from build123d import *
from build123d import SkipClean  # not in build123d's __all__

# Parameters (mm, degrees)
F1_DEPTH      = 2
F0_W          = 5.54
F0_H          = 25
F0_W_2        = 1.9
F0_W_3        = 2.5
F0_H_2        = 2.5
F2_DEPTH      = 5
F3_DEPTH      = 5
F4_DEPTH      = 7
F5_SIZE       = 7
F8_DEPTH      = 2
F9_SIZE       = 1.5
F10_SIZE      = 1.5
F11_SIZE      = 1.5
F12_R         = 8
F13_R         = 2
F14_T4_DEPTH  = 20.4300979278
F14_T10_DEPTH = 20.4300979278


# Not quite as in the source:
# - a fillet or chamfer that OpenCascade refuses, or shapes differently, is made with other operations: its cross-section is extruded or revolved along the edge and cut away or added
# - ends of sketch curves that miss each other by under 0.0002 mm in the source are joined
# - a feature names something its author has since deleted; it is built from what else it names


with BuildPart() as f1:
    # F0 (on Front) → F1 (new body)
    with BuildSketch(Plane.XZ):
        with BuildLine():
            Line((-25, 38.2831491688), (-4.67, 38.2831491688))
            Line((-4.67, 38.2831491688), (-4.67, 63.2831491688))
            Line((-4.67, 63.2831491688), (-12.45, 63.2831491688))
            Line((-12.45, 63.2831491688), (-12.45, 58.8677023414))
            ThreePointArc((-12.45, 58.8677023414), (-7.0483053281, 56.3311217715), (-4.85, 50.7831491688))
            ThreePointArc((-4.85, 50.7831491688), (-18.4979726027, 44.8814544969), (-13.45, 58.8677023414))
            Line((-13.45, 58.8677023414), (-13.45, 63.2831491688))
            Line((-13.45, 63.2831491688), (-25, 63.2831491688))
            Line((-25, 63.2831491688), (-25, 38.2831491688))
        make_face()
    extrude(amount=F1_DEPTH)



with BuildPart() as f1b:
    # F0 (on Front) → F1, piece 2 (new body)
    with BuildSketch(Plane.XZ):
        with BuildLine():
            Line((4.67, 38.2831491688), (25, 38.2831491688))
            Line((25, 38.2831491688), (25, 63.2831491688))
            Line((25, 63.2831491688), (13.45, 63.2831491688))
            Line((13.45, 63.2831491688), (13.45, 58.8677023414))
            ThreePointArc((13.45, 58.8677023414), (18.8516946719, 56.3311217715), (21.05, 50.7831491688))
            ThreePointArc((21.05, 50.7831491688), (7.4020273973, 44.8814544969), (12.45, 58.8677023414))
            Line((12.45, 58.8677023414), (12.45, 63.2831491688))
            Line((12.45, 63.2831491688), (4.67, 63.2831491688))
            Line((4.67, 63.2831491688), (4.67, 38.2831491688))
        make_face()
    extrude(amount=F1_DEPTH)


with BuildPart() as f1c:
    # F0 (on Front) → F1, piece 3 (new body)
    with BuildSketch(Plane.XZ):
        with Locations((0, 50.7831491688)):
            Rectangle(F0_W, F0_H)
        Polygon((2.77, -9.5068508312), (2.77, 38.2831491688), (-2.77, 38.2831491688), (-2.77, -9.5068508312), (-1.5, -9.5068508312), (-1.5, -0.9968508312), (1.5, -0.9968508312), (1.5, -9.5068508312), align=None)
    extrude(amount=F1_DEPTH)


with BuildPart() as f1_1:
    add(f1.part, clean=False)

    add(f1b.part)  # F2 merges F1b

    add(f1c.part)  # F2 merges F1c
    # F0 (on Front) → F2 (join)
    with BuildSketch(Plane.XZ):
        Polygon((-2.77, -9.5068508312), (-2.77, 38.2831491688), (-4.67, 38.2831491688), (-4.67, 0), (-4.67, -7.0068508312), (-4.67, -9.5068508312), align=None)
        Polygon((4.67, -7.0068508312), (4.67, 38.2831491688), (2.77, 38.2831491688), (2.77, -9.5068508312), (4.67, -9.5068508312), align=None)
        with Locations((3.72, 50.7831491688)):
            Rectangle(F0_W_2, F0_H)
        with Locations((-3.72, 50.7831491688)):
            Rectangle(F0_W_2, F0_H)
        with Locations((-5.92, -8.2568508312)):
            Rectangle(F0_W_3, F0_H_2)
        with Locations((5.92, -8.2568508312)):
            Rectangle(F0_W_3, F0_H_2)
    extrude(amount=F2_DEPTH)

    # F0 (on Front) → F3 (join)
    with BuildSketch(Plane.XZ):
        Polygon((1.5, -11.5068508312), (1.5, -9.5068508312), (1.5, -0.9968508312), (-1.5, -0.9968508312), (-1.5, -9.5068508312), (-1.5, -11.5068508312), align=None)
    extrude(amount=F3_DEPTH)

    # F4 (add): a face of the model
    f4_faces = [f1_1.faces().sort_by_distance(p)[0] for p in [
        (0, -5, -6.2518508312),
    ]]
    extrude(f4_faces, amount=F4_DEPTH)

    # F5
    f5_edges = [f1_1.edges().sort_by_distance(p)[0] for p in [
        (0, -12, -0.996851),
    ]]
    chamfer(f5_edges, length=F5_SIZE)

    # F7 (on face) → F8 (join)
    with BuildSketch(Plane(origin=(0, 0, -9.5068508312), x_dir=(1, 0, 0), z_dir=(0, 0, -1))):
        Polygon((15.0385206658, 12.000000352), (0.0385206658, 12.000000352), (-14.9614793342, 12.000000352), (-14.9614793342, 3.52e-07), (1.5, 3.52e-07), (1.5, 2), (2.77, 2), (2.77, 5), (7.17, 5), (7.17, 0), (15.0385206658, 3.52e-07), align=None)
        with BuildLine():
            ThreePointArc((-10.0064205471, 6.1577448677), (-12.5064205471, 8.6577448677), (-10.0064205471, 11.1577448677))
            Line((-10.0064205471, 11.1577448677), (10.0834618788, 11.1577448677))
            ThreePointArc((10.0834618788, 11.1577448677), (11.8512288318, 10.4255118207), (12.5834618788, 8.6577448677))
            ThreePointArc((12.5834618788, 8.6577448677), (11.8512288318, 6.8899779148), (10.0834618788, 6.1577448677))
            Line((10.0834618788, 6.1577448677), (-10.0064205471, 6.1577448677))
        make_face(mode=Mode.SUBTRACT)
        Polygon((1.5, 2), (1.5, 0), (7.17, 3.52e-07), (7.17, 5), (2.77, 5), (2.77, 2), align=None)
    with SkipClean():  # cleaning this boolean's faces spoils the solid; the shape is the same uncleaned
        extrude(amount=F8_DEPTH)

    # F9
    f9_edges = [f1_1.edges().sort_by_distance(p)[0] for p in [
        (15.038521, -12, -10.506851),
    ]]
    chamfer(f9_edges, length=F9_SIZE)

    # F10
    f10_edges = [f1_1.edges().sort_by_distance(p)[0] for p in [
        (-14.961479, -12, -10.506851),
    ]]
    chamfer(f10_edges, length=F10_SIZE)

    # F11
    f11_edges = [f1_1.edges().sort_by_distance(p)[0] for p in [
        (-14.961479, 0, -10.506851),
        (15.038521, 0, -10.506851),
    ]]
    chamfer(f11_edges, length=F11_SIZE)

    # F12
    f12_edges = [f1_1.edges().sort_by_distance(p)[0] for p in [
        (25, -1, 38.283149),
        (-25, -1, 38.283149),
        (-25, -1, 63.283149),
        (25, -1, 63.283149),
    ]]
    fillet(f12_edges, radius=F12_R)

    # F13
    f13_edges = [f1_1.edges().sort_by_distance(p)[0] for p in [
        (3.72, -5, 63.283149),
        (-3.72, -5, 63.283149),
    ]]
    fillet(f13_edges, radius=F13_R)

    # F14: chamfer of 3 on 2 edges, made by hand


with BuildPart() as f14_tool2:
    # F14_s3 → F14_t4 (new body)
    with BuildSketch(Plane.XZ.offset(-7.7150489639)):
        Polygon((4.17, -7.0068508312), (7.17, -10.0068508312), (7.17, -7.0068508312), align=None)
    extrude(amount=F14_T4_DEPTH)

    split(bisect_by=Plane.YZ.offset(4.67), keep=Keep.TOP)

    split(bisect_by=Plane.XY.offset(-9.5068508312), keep=Keep.TOP)


with BuildPart() as f1_2:
    add(f1_1.part, clean=False)

    # F14_t1: cut F14_tool2
    add(f14_tool2.part, mode=Mode.SUBTRACT)


with BuildPart() as f14_tool8:
    # F14_s9 → F14_t10 (new body)
    with BuildSketch(Plane.XZ.offset(-7.7150489639)):
        Polygon((-7.17, -10.0068508312), (-4.17, -7.0068508312), (-7.17, -7.0068508312), align=None)
    extrude(amount=F14_T10_DEPTH)

    split(bisect_by=Plane.YZ.offset(-4.67), keep=Keep.BOTTOM)

    split(bisect_by=Plane.XY.offset(-9.5068508312), keep=Keep.TOP)


with BuildPart() as f1_3:
    add(f1_2.part, clean=False)

    # F14_t7: cut F14_tool8
    add(f14_tool8.part, mode=Mode.SUBTRACT)


solid = f1_3.part
Model file for the job. Use its own axes, mm. A direction names the side the tool comes from. Coordinates: 2 decimals unless noted, no trailing zeros. Write each loop counter-clockwise with the first axis right and the second up, starting at its lowest first coordinate (ties: lowest second). Pieces come first, ordered by that corner, then holes. Notation, with made-up numbers: (-9, 6) - (4, 6) arc R24 ccw to (4, 24) - close; hole circle Ø4 at (14, -28.5). An arc over 180 degrees is marked (long way). Write each question's results on one line, items separated by ' | '. Start each with the question number.
1) Probe line 1 along Z through (x, y) = (12.95, -1.5); line 2 along X through (y, z) = (-0.75, 44); line 3 along X through (y, z) = (-3.5, 45.5). List the from-to ranges inside material, lowest first. Write a range as from..to.
2) Cut at C-C (z = -2). Write the cut outline in (x, y).
3) 3-axis set-ups, long thin cutter, end or side, ignore diameter. For faces 1 (the face through (6, -11.158, -10)), 2 (the face through (-11, -1, 38.283)), 3 (the face through (-2.77, -3, 26)), 4 (the face through (-12.45, -1, 61)), 5 (the face through (-14.2, -0.74, -10.49)): which of +Z, -Z, +X, -X, +Y, -Y reach the whole face in a straight line?
4) Cut at A-A (x = 11.5). Write the cut outline in (y, z), then the cut area to 3 significant figures.
5) Cut at D-D (z = 40). Write the cut outline in (x, y).
6) Mould opens along Y. For faces 6 (the face through (13.45, -1, 61)), 7 (the face through (-1.5, -6, -6)), 8 (the face through (0.021, -8.549, -4.546)) say: pulls with the +Y half, pulls with the -Y half, needs draft (parallel to the pull), parting line crosses it, or undercut.
7) Cut at B-B (z = 14). Write the cut outline in (x, y).
8) Flat gauge pins, fed straight in: P1, Ø2.5, axis at y = -3.5, z = 27.5, coming from the +X side; P2, Ø4.5, axis at x = -4, z = 13.5, coming from the -Y side; P3, Ø2.5, axis at y = -3.5, z = 10.5, coming from the -X side. Where does each tip first touch, or does it go through?
Returned:
1) line 1: -11.51..-9.51, 38.28..42.68 | line 2: -24.67..-17.38, -8.52..8.52, 17.38..24.67 | line 3: -4.67..-2.77, 2.77..4.67
2) outline: (-4.67, -5) - (-2.77, -5) - (-2.77, -2) - (-1.5, -2) - (-1.5, -6) - (1.5, -6) - (1.5, -2) - (2.77, -2) - (2.77, -5) - (4.67, -5) - (4.67, 0) - (-4.67, 0) - close
3) face 1: +Z, -Z | face 2: -X, +Y, -Y | face 3: +Z, -Y | face 4: +Z, +Y, -Y | face 5: -Z, -X, +Y
4) outline: (-12, -11.51) - (-10.72, -11.51) - (-10.72, -9.51) - (-12, -9.51) - close; (-6.6, -11.51) - (0, -11.51) - (0, -9.51) - (-6.6, -9.51) - close; (-2, 38.28) - (0, 38.28) - (0, 42.81) - (-2, 42.81) - close; (-2, 58.75) - (0, 58.75) - (0, 63.28) - (-2, 63.28) - close | area: 33.9 mm^2
5) outline: (-21.95, -2) - (-4.67, -2) - (-4.67, -5) - (-2.77, -5) - (-2.77, -2) - (2.77, -2) - (2.77, -5) - (4.67, -5) - (4.67, -2) - (21.95, -2) - (21.95, 0) - (-21.95, 0) - close
6) face 6: needs draft | face 7: undercut | face 8: pulls with the -Y half
7) outline: (-4.67, -5) - (-2.77, -5) - (-2.77, -2) - (2.77, -2) - (2.77, -5) - (4.67, -5) - (4.67, 0) - (-4.67, 0) - close
8) P1: x = 4.67 | P2: y = -5 | P3: x = -4.67
